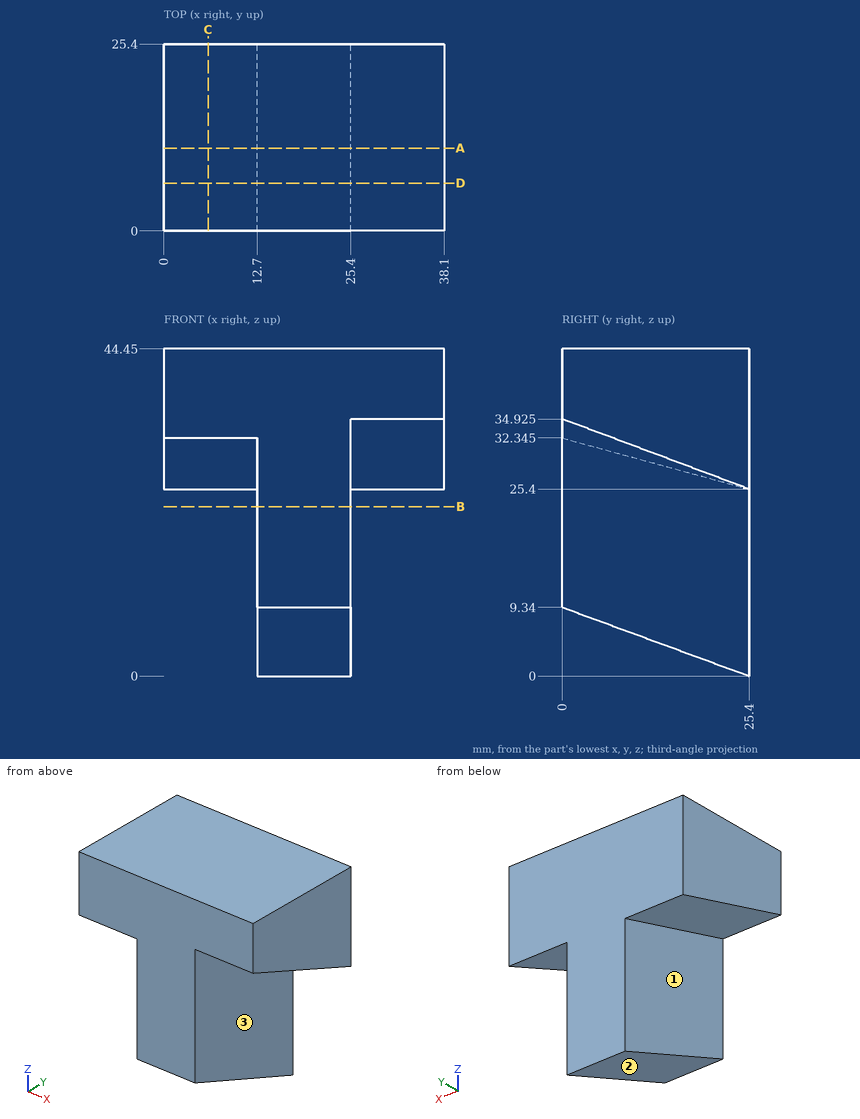
The figure shows three views and two pictorial views of one solid part (mm, origin at its lowest corner). Answer the questions. A direction names the side the tool comes from. Give positions to 0.01 mm unless a question says otherwise; leave off trailing zeros. Write each loop counter-clockwise with the first axis right and the second up, starting at its lowest first coordinate (ties: lowest second). Pieces come first, ordered by that corner, then holes. Notation, with made-up numbers: M -36.5,-6 L -32.5,-6 A22 cw -32.5,20 Z; hole C 86.25,-33 d7. An arc over 180 degrees is marked long. One line per item, written item: value. Start each with the question number.
(1) Find section B-B (z = 23). Determine the outline of the cut face in (x, y), plus the area to 3 significant figures.
(2) Find section D-D (y = 6.5). Determine the outline of the cut face in (x, z), plus the area to 4 significant figures.
(3) Find the intervals of material crossed by line 1 (X direction, y = 13.75, z = 29); line 2 (X direction, y = 5.25, z = 14); line 3 (Z direction, x = 14.5, y = 20.25), in increasing order.
(4) Find section C-C (x = 6). Determine the outline of the cut face in (y, z) (3 decimals).
(5) Find section A-A (y = 11.25). Determine the outline of the cut face in (x, z).
(6) Flat-ended cylindrical pins translate along their axes: pin 1 Ø6 at (y, z) = (13.5, 6) entering from -X; pin 2 Ø6 at (x, z) = (27.5, 27.5) entering from -Y; pin 3 Ø3 at (x, y) = (26.5, 5.5) entering from -Z; pin 4 Ø3 at (x, y) = (18, 4) entering from -Z. Find the tip coordinate at first contact, or state that the pin passes through.
(7) A tool of negligible diameter and unlimited length cuts with its end or side. For the marked faces 1, 2 and 3, from which of +Z, -Z, +X, -X, +Y, -Y can it reach the whole face along a straight path? Write none if from no direction.
Results below:
1. outline: M 12.7,0 L 25.4,0 L 25.4,25.4 L 12.7,25.4 Z
1. area: 323 mm^2
2. outline: M 0,30.57 L 12.7,30.57 L 12.7,6.95 L 25.4,6.95 L 25.4,32.49 L 38.1,32.49 L 38.1,44.45 L 0,44.45 Z
2. area: 804.5 mm^2
3. line 1: x = 0 to 25.4
3. line 2: x = 12.7 to 25.4
3. line 3: z = 1.89 to 44.45
4. outline: M 0,32.345 L 25.4,25.4 L 25.4,44.45 L 0,44.45 Z
5. outline: M 0,29.27 L 12.7,29.27 L 12.7,5.2 L 25.4,5.2 L 25.4,30.71 L 38.1,30.71 L 38.1,44.45 L 0,44.45 Z
6. pin 1: stops at x = 12.7
6. pin 2: stops at y = 0
6. pin 3: stops at z = 6.94
6. pin 4: stops at z = 7.32
7. face 1: -Z, -X, -Y
7. face 2: -Z, +X, -X, -Y
7. face 3: -Z, +X, -Y
